The model under review builds one solid part; all positions refer to its coordinate system, in mm. Face numbers are marked on the shaded views. A direction names the side the tool comes from. Give positions to 0.01 mm unless a question says otherwise; leave off trailing zeros. Loops run counter-clockwise (first coordinate to the right, second up) from the corner with the lowest first, then second, coordinate; pieces in that order, holes last. Notation, with made-up numbers: (72.5, -38.5) -> (121.5, -38.5) arc R25 cw to (121.5, -17.5) -> close; hole circle Ø11 at (-21.75, 75). An arc over 180 degrees is marked (long way). Write each question's results on one line, items separated by ' | '. Start each with the question number.
Q1. Wall thickness on L1, parallel to X at y = 0, z = 7.25; L2, parallel to X at y = -9.75, z = 18.5: over which ranges is each line inside the solid? List them lowest first. Write a range as [from, to].
Q2. Insertion check: pin 1 Ø4.5 at (x, y) = (0, 0) entering from -Z; pin 2 Ø2 at (x, y) = (-10, 3.5) entering from -Z; pin 3 Ø1.1 at (y, z) = (-10, 14.5) entering from -X; pin 4 Ø10 at (x, y) = (-2.5, -8) entering from +Z. Each pin has a flat end and moves straight along its axis. Give the tip position at first contact, or say it passes through.
Q3. We need section B-B (z = 18.75). Write out the cut boundary in (x, y).
Q4. We need section D-D (z = 8). Write out the cut boundary in (x, y).
Q5. We need section A-A (y = 0). Write out the cut boundary in (x, z).
Q6. Machinability: for the marked faces 1, 2 and 3, which of the approach directions +Z, -Z, +X, -X, +Y, -Y give a long, thin tool a straight path to every point of the face, cutting with its end or side? Answer none if there is none.
Autodesk Inventor part; units mm, degrees
ref_plane "YZ Plane" through (0, 0, 0) normal (1, 0, 0) x (0, 1, 0)
ref_plane "XZ Plane" through (0, 0, 0) normal (0, 1, 0) x (-1, 0, 0)
ref_plane "XY Plane" through (0, 0, 0) normal (0, 0, 1) x (1, 0, 0)
sketch "Sketch1" plane through (0, 0, 0) normal (0, 0, 1) x (1, 0, 0)
  line L0 (-14.25, -14.25) -> (14.25, -14.25)
  line L1 (14.25, -14.25) -> (14.25, 14.25)
  line L2 (14.25, 14.25) -> (-14.25, 14.25)
  line L3 (-14.25, 14.25) -> (-14.25, -14.25)
  line L4 (-14.25, -14.25) -> (14.25, 14.25) construction
  line L5 (14.25, -14.25) -> (-14.25, 14.25) construction
  point P0 (0, 0)
  dimension "d0" = 28.5
  dimension "d1" = 28.5
extrude "Extrusion1" add sketch "Sketch1" along normal blind 11.5
sketch "Sketch2" plane through (0, 0, 11.5) normal (0, 0, 1) x (1, 0, 0)
  line L0 (-10.15, 4.1) -> (-9.15, 4.1)
  line L1 (-9.15, 4.1) -> (-9.15, 10.4)
  line L2 (-9.15, 10.4) -> (-10.15, 10.4)
  line L3 (-10.15, 10.4) -> (-10.15, 4.1)
  line L4 (-10.15, -10.4) -> (-9.15, -10.4)
  line L5 (-9.15, -10.4) -> (-9.15, -4.1)
  line L6 (-9.15, -4.1) -> (-10.15, -4.1)
  line L7 (-10.15, -4.1) -> (-10.15, -10.4)
  line L8 (3.85, -10.4) -> (10.15, -10.4)
  line L9 (10.15, -10.4) -> (10.15, -9.4)
  line L10 (10.15, -9.4) -> (3.85, -9.4)
  line L11 (3.85, -9.4) -> (3.85, -10.4)
  line L12 (9.15, 10.4) -> (10.15, 10.4)
  line L13 (10.15, 10.4) -> (10.15, 4.1)
  line L14 (10.15, 4.1) -> (9.15, 4.1)
  line L15 (9.15, 4.1) -> (9.15, 10.4)
  line L16 (-9.15, 4.1) -> (-9.15, -4.1) construction
  line L17 (-9.15, 10.4) -> (9.15, 10.4) construction
  point P0 (0, 0)
  point P1 (-9.15, 0)
  point P2 (0, 10.4)
  dimension "d4" = 1
  dimension "d5" = 1
  dimension "d6" = 1
  dimension "d7" = 6.3
  dimension "d8" = 6.3
  dimension "d9" = 6.3
  dimension "d10" = 8.2
  dimension "d11" = 13
extrude "Extrusion2" add sketch "Sketch2" along normal blind 10
sketch "Sketch3" plane through (0, 0, 11.5) normal (0, 0, 1) x (1, 0, 0)
  point P0 (0, 0)
  point P1 (0, 0)
hole "Hole1" at (0, 0, 11.5) direction (0, 0, -1) diameter 5.5 end through all
fillet "Fillet1" radius 1 4 edges at (14.25, 14.25, 5.75) (-14.25, 14.25, 5.75) (-14.25, -14.25, 5.75) (14.25, -14.25, 5.75)
properties part number "Gleichrichter"
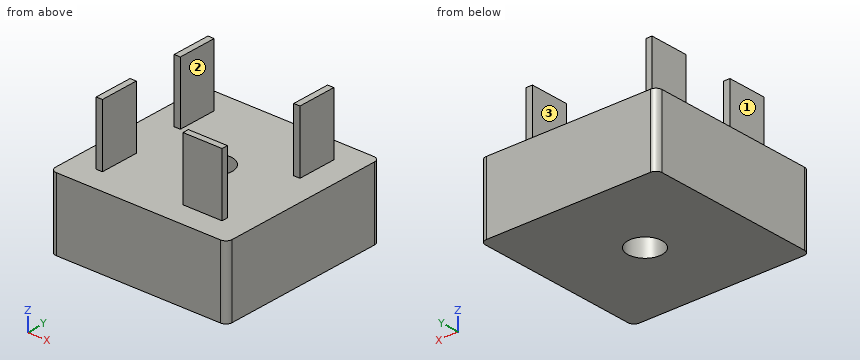
Output:
1) L1: [-14.25, -2.75], [2.75, 14.25] | L2: [-10.15, -9.15], [3.85, 10.15]
2) pin 1: through | pin 2: z = 0 | pin 3: x = -10.15 | pin 4: z = 11.5
3) outline: (-10.15, -10.4) -> (-9.15, -10.4) -> (-9.15, -4.1) -> (-10.15, -4.1) -> close; (-10.15, 4.1) -> (-9.15, 4.1) -> (-9.15, 10.4) -> (-10.15, 10.4) -> close; (3.85, -10.4) -> (10.15, -10.4) -> (10.15, -9.4) -> (3.85, -9.4) -> close; (9.15, 4.1) -> (10.15, 4.1) -> (10.15, 10.4) -> (9.15, 10.4) -> close
4) outline: (-14.25, -13.25) arc R1 ccw to (-13.25, -14.25) -> (13.25, -14.25) arc R1 ccw to (14.25, -13.25) -> (14.25, 13.25) arc R1 ccw to (13.25, 14.25) -> (-13.25, 14.25) arc R1 ccw to (-14.25, 13.25) -> close; hole circle Ø5.5 at (0, 0)
5) outline: (-14.25, 0) -> (-2.75, 0) -> (-2.75, 11.5) -> (-14.25, 11.5) -> close; (2.75, 0) -> (14.25, 0) -> (14.25, 11.5) -> (2.75, 11.5) -> close
6) face 1: +Z, -X, +Y, -Y | face 2: +Z, +Y, -Y | face 3: +Z, +Y
